```python
from build123d import *

# Parameters (mm, degrees)
MODEL_R         = 1.6
MODEL_R_2       = 18
MODEL_R_3       = 4
MODEL_R_4       = 2
EXTRUDE_1_DEPTH = 3


with BuildPart() as part:
    # Model → 凸台-拉伸1 (new body)
    with BuildSketch(Plane.XY):
        with BuildLine():
            Line((-69.018143336, -8.419028309), (-9.766132819, 45.183203451))
            ThreePointArc((-9.766132819, 45.183203451), (-1.715728752, 48.284271248), (6.334675314, 45.183203451))
            Line((6.334675314, 45.183203451), (65.586685831, -8.419028309))
            ThreePointArc((65.586685831, -8.419028309), (69.783384512, -26.035623827), (54.852813742, -36.284271247))
            Line((54.852813742, -36.284271247), (-58.284271247, -36.284271247))
            ThreePointArc((-58.284271247, -36.284271247), (-73.214842017, -26.035623827), (-69.018143336, -8.419028309))
        make_face()
        with Locations((5.715728753, -25.784271247)):
            Circle(MODEL_R, mode=Mode.SUBTRACT)
        Circle(MODEL_R_2, mode=Mode.SUBTRACT)
        with Locations((-58.284271248, -20.284271247)):
            Circle(MODEL_R_3, mode=Mode.SUBTRACT)
        with Locations((-1.715728753, 36.284271247)):
            Circle(MODEL_R_3, mode=Mode.SUBTRACT)
        with Locations((-22.284271247, -25.784271247)):
            Circle(MODEL_R, mode=Mode.SUBTRACT)
        with Locations((-34.284271247, -25.784271247)):
            Circle(MODEL_R, mode=Mode.SUBTRACT)
        with Locations((17.715728753, -25.784271247)):
            Circle(MODEL_R, mode=Mode.SUBTRACT)
        with Locations((-66.769552622, -11.798989873)):
            Circle(MODEL_R_4, mode=Mode.SUBTRACT)
        with Locations((-49.798989873, -11.798989873)):
            Circle(MODEL_R_4, mode=Mode.SUBTRACT)
        with Locations((-49.798989873, -28.769552622)):
            Circle(MODEL_R_4, mode=Mode.SUBTRACT)
        with Locations((-66.769552622, -28.769552622)):
            Circle(MODEL_R_4, mode=Mode.SUBTRACT)
    extrude(amount=EXTRUDE_1_DEPTH)


solid = part.part
```
Work out the finished part from the listing and answer in its coordinate system (mm). Give positions to 0.01 mm unless a question says otherwise; leave off trailing zeros. Order: outer loops, then holes, each group sorted by start corner. A loop starts at its lowest first (then second) coordinate and runs counter-clockwise, first axis right, second up.
1. Section A-A, the plane x = 11 is taken. Determine the outline of the cut face in (y, z), and give its area (3 significant figures).
Result sheet:
outline: (-36.28, 0) - (-14.25, 0) - (-14.25, 3) - (-36.28, 3) - close; (14.25, 0) - (40.96, 0) - (40.96, 3) - (14.25, 3) - close
area: 146 mm2
2. The mould has two halves that part along Y. Classify faces 1 (the cylindrical face through (-1.839, 48.284, 1.479)), 2 (the cylindrical face through (-47.951, -29.536, 1.479)), 3 (the flat face through (15, -12, 3)): released by +Y, released by -Y, zero draft, split by the parting line, or undercut.
Result sheet:
face 1: released by +Y
face 2: undercut
face 3: zero draft
3. Each of these flat-tipped pins is pushed along its axis until it touches: P1, Ø3.5, axis at x = -66.77, y = -11.8, coming from the -Z side; P2, Ø1.5, axis at y = 27, z = 0.5, coming from the +X side; P3, Ø1, axis at y = 20, z = 1.5, coming from the -X side. Where does it stop, or does it pass through?
Result sheet:
P1: passes through
P2: stops at x = 27.26
P3: stops at x = -38.16
4. Section C-C, the plane z = 1.75 is taken. Give the number of separate pieces and of enclosed holes in the cut face, and give its area (3 significant figures).
Result sheet:
separate pieces: 1
enclosed holes: 11
area: 6,770 mm2
5. Section D-D, the plane x = 50.5 is taken. Determine the outline of the cut face in (y, z).
Result sheet:
outline: (-36.28, 0) - (5.23, 0) - (5.23, 3) - (-36.28, 3) - close
6. Section B-B, the plane y = 6.5 is taken. Determine the outline of the cut face in (x, z).
Result sheet:
outline: (-52.53, 0) - (-16.79, 0) - (-16.79, 3) - (-52.53, 3) - close; (16.79, 0) - (49.1, 0) - (49.1, 3) - (16.79, 3) - close
7. Straight lines are drawn through the part: L1, parallel to X at y = -11, z = 0.25; L2, parallel to Y at x = 15.5, z = 1.5; L3, parallel to X at y = -29, z = 0.55. For each, find the intervals that lie inside material, in ascending order.
Result sheet:
L1: x = -71.32 to -68.6, -64.94 to -51.63, -47.97 to -14.25, 14.25 to 67.88
L2: y = -36.28 to -9.15, 9.15 to 36.89
L3: x = -71.7 to -68.76, -64.78 to -51.79, -47.81 to 68.27
